Part model, mm, in its own coordinate system. A direction names the side the tool comes from. Give positions to 0.01 mm unless a question says otherwise; leave off trailing zeros. Order: outer loops, then holes, each group sorted by start corner. A loop starts at its lowest first (then second) coordinate and runs counter-clockwise, first axis right, second up.
Autodesk Inventor part; units mm, degrees
ref_plane "YZ Plane" through (0, 0, 0) normal (1, 0, 0) x (0, 1, 0)
ref_plane "XZ Plane" through (0, 0, 0) normal (0, 1, 0) x (-1, 0, 0)
ref_plane "XY Plane" through (0, 0, 0) normal (0, 0, 1) x (1, 0, 0)
ref_plane "Arbeitsebene1" through (0, 0, 0) normal (0, 0, 1) x (1, 0, 0)
sketch "Skizze1" plane through (0, 0, 0) normal (0, 0, 1) x (1, 0, 0)
  line L0 (6, 17.9) -> (7, 16.9)
  line L1 (3.1, 17.9) -> (6, 17.9)
  line L2 (3.1, 14) -> (3.1, 17.9)
  line L3 (3.5, 14) -> (3.1, 14)
  line L4 (3.5, 10) -> (3.5, 14)
  line L5 (6.4, 10) -> (3.5, 10)
  line L6 (6.4, -11.4) -> (6.4, 10)
  line L7 (3.8, -11.4) -> (6.4, -11.4)
  line L8 (3.8, -14.4) -> (3.8, -11.4)
  line L9 (1.3, -14.4) -> (3.8, -14.4)
  line L10 (1.3, -13.4) -> (1.3, -14.4)
  line L11 (-0.7, -13.4) -> (1.3, -13.4)
  line L12 (-0.7, -14.4) -> (-0.7, -13.4)
  line L13 (-6.9, -14.4) -> (-5.1, -14.4)
  line L14 (-4.1, -13.4) -> (-4.1, -14.4)
  line L15 (-5.1, -13.4) -> (-4.1, -13.4)
  line L16 (-5.1, -14.4) -> (-5.1, -13.4)
  line L17 (-6.9, -17.9) -> (-6.9, -14.4)
  line L18 (6, -17.9) -> (-6.9, -17.9)
  line L19 (7, -16.9) -> (6, -17.9)
  line L20 (7, 16.9) -> (7, -16.9)
  line L21 (6, 17.9) -> (7, 16.9)
  line L22 (3.1, 17.9) -> (6, 17.9)
  line L23 (3.1, 14) -> (3.1, 17.9)
  line L24 (3.5, 14) -> (3.1, 14)
  line L25 (3.5, 10) -> (3.5, 14)
  line L26 (6.4, 10) -> (3.5, 10)
  line L27 (6.4, -11.4) -> (6.4, 10)
  line L28 (3.8, -11.4) -> (6.4, -11.4)
  line L29 (3.8, -14.4) -> (3.8, -11.4)
  line L30 (1.3, -14.4) -> (3.8, -14.4)
  line L31 (1.3, -13.4) -> (1.3, -14.4)
  line L32 (-0.7, -13.4) -> (1.3, -13.4)
  line L33 (-0.7, -14.4) -> (-0.7, -13.4)
  line L34 (-6.9, -14.4) -> (-5.1, -14.4)
  line L35 (-4.1, -13.4) -> (-4.1, -14.4)
  line L36 (-5.1, -13.4) -> (-4.1, -13.4)
  line L37 (-5.1, -14.4) -> (-5.1, -13.4)
  line L38 (-6.9, -17.9) -> (-6.9, -14.4)
  line L39 (6, -17.9) -> (-6.9, -17.9)
  line L40 (7, -16.9) -> (6, -17.9)
  line L41 (7, 16.9) -> (7, -16.9)
  line L42 (-9.8, -17.9) -> (-10.8, -16.9)
  line L43 (-6.9, -17.9) -> (-9.8, -17.9)
  line L44 (-6.9, -14) -> (-6.9, -17.9)
  line L45 (-7.3, -14) -> (-6.9, -14)
  line L46 (-7.3, -10) -> (-7.3, -14)
  line L47 (-10.2, -10) -> (-7.3, -10)
  line L48 (-10.2, 11.4) -> (-10.2, -10)
  line L49 (-7.6, 11.4) -> (-10.2, 11.4)
  line L50 (-7.6, 14.4) -> (-7.6, 11.4)
  line L51 (-5.1, 14.4) -> (-7.6, 14.4)
  line L52 (-5.1, 13.4) -> (-5.1, 14.4)
  line L53 (-3.1, 13.4) -> (-5.1, 13.4)
  line L54 (-3.1, 14.4) -> (-3.1, 13.4)
  line L55 (3.1, 14.4) -> (1.3, 14.4)
  line L56 (0.3, 13.4) -> (0.3, 14.4)
  line L57 (1.3, 13.4) -> (0.3, 13.4)
  line L58 (1.3, 14.4) -> (1.3, 13.4)
  line L59 (3.1, 17.9) -> (3.1, 14.4)
  line L60 (-9.8, 17.9) -> (3.1, 17.9)
  line L61 (-10.8, 16.9) -> (-9.8, 17.9)
  line L62 (-10.8, -16.9) -> (-10.8, 16.9)
  arc A0 (5.1, -4.25) -> (6.1, -3.25) centre (5.1, -3.25) ccw construction
  line L63 (6.1, 2.25) -> (6.1, -3.25) construction
  arc A1 (6.1, 2.25) -> (5.1, 3.25) centre (5.1, 2.25) ccw construction
  line L64 (3.3, 3.25) -> (5.1, 3.25) construction
  line L65 (3.3, 3.25) -> (3.3, -4.25) construction
  line L66 (3.3, -4.25) -> (5.1, -4.25) construction
  arc A2 (-8.9, 4.25) -> (-9.9, 3.25) centre (-8.9, 3.25) ccw construction
  line L67 (-9.9, -2.25) -> (-9.9, 3.25) construction
  arc A3 (-9.9, -2.25) -> (-8.9, -3.25) centre (-8.9, -2.25) ccw construction
  line L68 (-7.1, -3.25) -> (-8.9, -3.25) construction
  line L69 (-7.1, -3.25) -> (-7.1, 4.25) construction
  line L70 (-7.1, 4.25) -> (-8.9, 4.25) construction
  line L71 (3, -4.55) -> (3, 3.55)
  line L72 (3, 3.55) -> (5.1, 3.55)
  arc A4 (6.4, 2.25) -> (5.1, 3.55) centre (5.1, 2.25) ccw
  line L73 (6.4, 2.25) -> (6.4, -3.25)
  arc A5 (5.1, -4.55) -> (6.4, -3.25) centre (5.1, -3.25) ccw
  line L74 (5.1, -4.55) -> (3, -4.55)
  arc A6 (-10.2, -2.25) -> (-8.9, -3.55) centre (-8.9, -2.25) ccw
  line L75 (-10.2, -2.25) -> (-10.2, 3.25)
  arc A7 (-8.9, 4.55) -> (-10.2, 3.25) centre (-8.9, 3.25) ccw
  line L76 (-8.9, 4.55) -> (-6.8, 4.55)
  line L77 (-6.8, 4.55) -> (-6.8, -3.55)
  line L78 (-6.8, -3.55) -> (-8.9, -3.55)
  circle A8 centre (4.7, -15.8) radius 1.4
  circle A9 centre (4.7, -15.8) radius 1.4
  circle A10 centre (-8.5, 15.8) radius 1.4
  circle A11 centre (-4.1, -15.8) radius 1.4
  circle A12 centre (-4.1, -15.8) radius 1.4
  line L79 (-4.1, -14.4) -> (-0.7, -14.4)
  circle A13 centre (-4.1, -15.8) radius 1.4
  circle A14 centre (-4.1, -15.8) radius 1.4
  line L80 (-4.1, -14.4) -> (-0.7, -14.4)
  circle A15 centre (0.3, 15.8) radius 1.4
  circle A16 centre (0.3, 15.8) radius 1.4
  line L81 (0.3, 14.4) -> (-3.1, 14.4)
  point P0 (0, 0)
  point P1 (-2.4, -14.4)
  point P2 (-2.5, -14.4)
  point P3 (-1.4, 14.4)
  point P4 (-1.3, 14.4)
  dimension "d0" = 0.3
  dimension "d1" = 0.3
extrude "Extrusion1" add sketch "Skizze1" along normal blind 3 contours A11 | L0 L20 L19 L18 L17 L13 L16 L15 L14 L79 L12 L11 L10 L9 L8 L7 L6 L5 L4 L3 L2 L1 | A15 | L2 L55 L58 L57 L56 L81 L54 L53 L52 L51 L50 L49 L48 L47 L46 L45 L44 L17 L43 L42 L62 L61 L60 | L2 L3 L4 L5 L6 A4 L72 L71 L74 A5 L7 L8 L9 L10 L11 L12 L79 L14 L15 L16 L13 L44 L45 L46 L47 L48 A6 L78 L77 L76 A7 L49 L50 L51 L52 L53 L54 L81 L56 L57 L58 L55 | A8 | A10
sketch "Skizze2" plane through (0, 0, 3) normal (0, 0, 1) x (1, 0, 0)
  point P0 (0, 0)
sketch "Skizze3" plane through (0, 0, 3) normal (0, 0, 1) x (1, 0, 0)
  circle A0 centre (-8.5, 15.8) radius 1.4
  circle A1 centre (0.3, 15.8) radius 1.4
  circle A2 centre (4.7, -15.8) radius 1.4
  circle A3 centre (-4.1, -15.8) radius 1.4
  point P0 (0, 0)
hole "Bohrung1" at (0.3, 15.8, 3) at (4.7, -15.8, 3) at (-4.1, -15.8, 3) at (-8.5, 15.8, 3) direction (0, 0, -1) diameter 2.8 depth 12 tip angle 118 counterbore diameter 5.5 counterbore depth 1
chamfer "Fase1" distance 2 angle 45 12 edges at (6.0192, 3.1692, 3) (6.4, -0.5, 3) (6.0192, -4.1692, 3) (4.05, -4.55, 3) (4.05, 3.55, 3) (3, -0.5, 3) (-6.8, 0.5, 3) (-9.8192, 4.1692, 3) (-7.85, 4.55, 3) (-10.2, 0.5, 3) (-9.8192, -3.1692, 3) (-7.85, -3.55, 3)
properties part number "02_Camera_Module_Lid_v0"
Item 1: Band-saw the part on A-A on y = 15.8. List the corners of the cut face in (x, z), plus the area to 4 significant figures.
Item 2: Pull direction X, two halves, no side cores. Call faces 4 (the face through (6.5, -17.4, 1)), 5 (the face through (-2, 0, 0)), 6 (the face through (-6.8, 0.6, 0.5)): released by +X, released by -X, zero draft, split by the parting line, or undercut.
Item 3: Which spindle directions (+Z, -Z, +X, -X, +Y, -Y) get a long thin tool onto all of the face, cutting with end or side? Do faces 1 (the face through (-10.8, 0, 1)), 2 (the face through (-9.81, -3.18, 0.49)), 3 (the face through (-7.33, 5.54, 1.99)). Say none if no direction does.
Item 4: Band-saw the part on B-B on x = 0.3. List the corners of the cut face in (y, z).
Item 5: Band-saw the part on C-C on x = -8.5. List the corners of the cut face in (y, z).
Item 6: Drill centre lines: probe 1 along X at (y, z) = (15.8, 0.4); probe 2 along X at (y, z) = (15.8, 2.5); probe 3 along X at (y, z) = (-15.8, 2.65). Where is each one in solid material? Low to high.
Item 7: Drop flat-ended pins along their axis: P1, Ø4, axis at x = -8, y = 15.5, coming from the +Z side; P2, Ø1.5, axis at x = -7, y = -1, coming from the +Z side. Give the stop position or say it passes through.
Working result:
1. outline: (-10.8, 0) - (-9.9, 0) - (-9.9, 2) - (-10.8, 2) - close; (-7.1, 0) - (-1.1, 0) - (-1.1, 2) - (-2.45, 2) - (-2.45, 3) - (-5.75, 3) - (-5.75, 2) - (-7.1, 2) - close; (1.7, 0) - (7, 0) - (7, 3) - (3.05, 3) - (3.05, 2) - (1.7, 2) - close
1. area: 31.65 mm2
2. face 4: released by +X
2. face 5: zero draft
2. face 6: undercut
3. face 1: +Z, -Z, -X, +Y, -Y
3. face 2: +Z, -Z
3. face 3: +Z
4. outline: (-17.9, 0) - (14.4, 0) - (14.4, 2) - (13.05, 2) - (13.05, 3) - (-17.9, 3) - close; (17.2, 0) - (17.9, 0) - (17.9, 2) - (17.2, 2) - close
5. outline: (-17.9, 0) - (-3.55, 0) - (-3.55, 1) - (-5.55, 3) - (-17.9, 3) - close; (4.55, 0) - (14.4, 0) - (14.4, 2) - (13.05, 2) - (13.05, 3) - (6.55, 3) - (4.55, 1) - close; (17.2, 0) - (17.9, 0) - (17.9, 2) - (17.2, 2) - close
6. probe 1: x = -10.8 to -9.9, -7.1 to -1.1, 1.7 to 7
6. probe 2: x = -5.75 to -2.45, 3.05 to 7
6. probe 3: x = -10.8 to -6.85, -1.35 to 1.95
7. P1: stops at z = 2
7. P2: stops at z = 1.55
